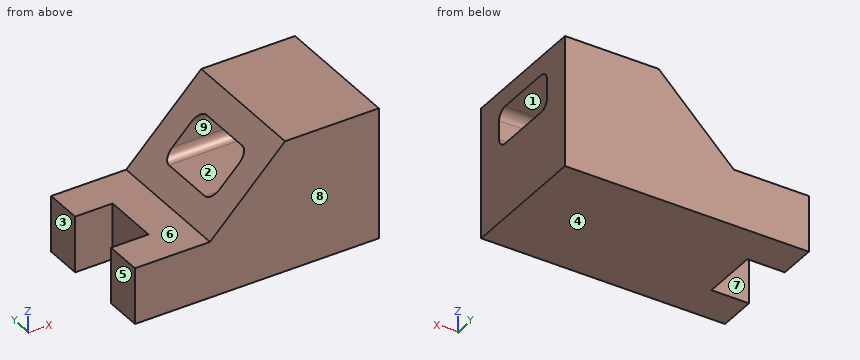
```python
from build123d import *

# Parameters (mm, degrees)
F1_DEPTH = 700
F3_DEPTH = 1300.001
F4_W     = 200
F4_H     = 300
F5_DEPTH = 300.001


with BuildPart() as f1:
    # F0 (on Front) → F1 (new body)
    with BuildSketch(Plane.XZ):
        Polygon((650, 350), (150, 350), (-250, -50), (-650, -50), (-650, -350), (650, -350), align=None)
    extrude(amount=F1_DEPTH)

    # F2 (on face) → F3 (cut, through all)
    with BuildSketch(Plane.YZ.offset(650)):
        with BuildLine():
            Line((-200, 250), (-500, 250))
            ThreePointArc((-500, 250), (-535.355339, 235.355339), (-550, 200))
            Line((-550, 200), (-550, 100))
            ThreePointArc((-550, 100), (-535.355339, 64.644661), (-500, 50))
            Line((-500, 50), (-200, 50))
            ThreePointArc((-200, 50), (-164.644661, 64.644661), (-150, 100))
            Line((-150, 100), (-150, 200))
            ThreePointArc((-150, 200), (-164.644661, 235.355339), (-200, 250))
        make_face()
    extrude(amount=-F3_DEPTH, mode=Mode.SUBTRACT)

    # F4 (on face) → F5 (cut, through all)
    with BuildSketch(Plane.XY.offset(-50)):
        with Locations((-550, -350)):
            Rectangle(F4_W, F4_H)
    extrude(amount=-F5_DEPTH, mode=Mode.SUBTRACT)


solid = f1.part
```
Could you check a few things on this model? Use its own coordinates, in mm. Face numbers are marked on the shaded views. A direction names the side the tool comes from. Round coordinates to 2 decimals unless told otherwise and drop trailing zeros. Write each loop counter-clockwise with the first axis right and the second up, starting at its lowest first coordinate (ties: lowest second). Pieces come first, ordered by that corner, then holes. Notation, with made-up numbers: M 70.25,-12 L 89.25,-12 A22 ccw 89.25,12 Z; hole C 9,0 d9. An arc over 180 degrees is marked long. Write each question's results on one line, items separated by ' | '. Start each with the question number.
1. Thinking about a two-plate mould opening in Z: for the marked faces 1, 2, 3 and 4, which applies, +Z half, -Z half, draft (parallel to the pull), parting line (faces both ways), or undercut?
2. Imagine slicing it at C-C on x = 413. List the corners of the cut face in (y, z) for me.
3. Imagine slicing it at D-D on z = -144.5. List the corners of the cut face in (x, y) for me, and give its area (3 significant figures).
4. I'm going to push flat-ended pins straight in: pin 1 Ø3 at (x, y) = (-215.5, -224) entering from +Z; pin 2 Ø1.5 at (y, z) = (-273, -1) entering from -X. Where does each tip first touch, or does it pass through?
5. Imagine slicing it at B-B on x = -536. List the corners of the cut face in (y, z) for me.
6. I need wall thicknesses on L1, parallel to Z at x = 363.5, y = -459; L2, parallel to Z at x = -367, y = -125; L3, parallel to X at y = -497.5, z = -88. Which ranges of each line are inside material? Lowest first, please. Write a range as from..to.
7. On a 3-axis mill with a long thin cutter (end or side, diameter ignored), from which of +Z, -Z, +X, -X, +Y, -Y can I reach the whole of each face in a straight line? I mean the marked faces 5, 6, 7, 8 and 9. Say none if no direction works.
8. Imagine slicing it at A-A on y = -291.5. List the corners of the cut face in (x, z) for me.
Result sheet:
1) face 1: undercut | face 2: undercut | face 3: draft | face 4: -Z half
2) outline: M -700,-350 L 0,-350 L 0,350 L -700,350 Z; hole M -550,100 A50 ccw -500,50 L -200,50 A50 ccw -150,100 L -150,200 A50 ccw -200,250 L -500,250 A50 ccw -550,200 Z
3) outline: M -650,-700 L 650,-700 L 650,0 L -650,0 L -650,-200 L -450,-200 L -450,-500 L -650,-500 Z | area: 850,000 mm^2
4) pin 1: stops at z = -14 | pin 2: stops at x = -201.75
5) outline: M -700,-350 L -500,-350 L -500,-50 L -700,-50 Z; M -200,-350 L 0,-350 L 0,-50 L -200,-50 Z
6) L1: z = -350..50, 250..350 | L2: z = -350..-50 | L3: x = -450..650
7) face 5: +Z, -Z, -X, +Y, -Y | face 6: +Z, -X, +Y, -Y | face 7: +Z, -Z, -X | face 8: +Z, -Z, +X, -X, -Y | face 9: +X, -X
8) outline: M -450,-350 L 650,-350 L 650,50 L -150,50 L -250,-50 L -450,-50 Z; M 50,250 L 650,250 L 650,350 L 150,350 Z
